Read the model definition and answer for the solid it produces. Units are mm, in the model's axes. Face numbers are marked on the shaded views. Give positions to 0.01 mm unless a question says otherwise; leave off trailing zeros. Loops run counter-clockwise (first coordinate to the right, second up) from the corner with the lowest first, then second, coordinate; pieces in that order, holes last. Notation, with made-up numbers: (43, 65.5) -> (99, 65.5) arc R7 ccw to (99, 71.5) -> close; hole circle Ø2 at (8, 66.25). An arc over 180 degrees is marked (long way). Return JSON: item names as keys, results as strings. Group by question number.
Autodesk Inventor part; units mm, degrees
ref_plane "YZ Plane" through (0, 0, 0) normal (1, 0, 0) x (0, 1, 0)
ref_plane "XZ Plane" through (0, 0, 0) normal (0, 1, 0) x (-1, 0, 0)
ref_plane "XY Plane" through (0, 0, 0) normal (0, 0, 1) x (1, 0, 0)
sketch "Sketch1" plane through (0, 0, 0) normal (0, 0, 1) x (1, 0, 0)
  line L0 (-66.75, 41.75) -> (66.75, 41.75)
  line L1 (66.75, 41.75) -> (66.75, -41.75)
  line L2 (66.75, -41.75) -> (-66.75, -41.75)
  line L3 (-66.75, -41.75) -> (-66.75, 41.75)
  line L4 (-66.75, 41.75) -> (66.75, -41.75) construction
  line L5 (66.75, 41.75) -> (-66.75, -41.75) construction
  circle A0 centre (-63.75, 38.75) radius 1.5
  circle A1 centre (63.75, 38.75) radius 1.5
  circle A2 centre (63.75, -38.75) radius 1.5
  circle A3 centre (-63.75, -38.75) radius 1.5
  point P0 (0, 0)
  dimension "d0" = 133.5
  dimension "d1" = 83.5
  dimension "d2" = 3
  dimension "d3" = 3
  dimension "d4" = 3
  dimension "d5" = 3
  dimension "d6" = 3
  dimension "d7" = 3
  dimension "d8" = 3
  dimension "d9" = 3
  dimension "d10" = 3
  dimension "d11" = 3
  dimension "d12" = 3
  dimension "d13" = 3
extrude "Extrusion1" add sketch "Sketch1" along normal blind 1.75
fillet "Fillet1" radius 3 4 edges at (66.75, 41.75, 0.875) (-66.75, 41.75, 0.875) (66.75, -41.75, 0.875) (-66.75, -41.75, 0.875)
sketch "Sketch2" plane through (0, 0, 1.75) normal (0, 0, 1) x (1, 0, 0)
  line L0 (-59.5, 37.75) -> (59.5, 37.75)
  line L1 (59.5, 37.75) -> (59.5, -39.75)
  line L2 (59.5, -39.75) -> (-59.5, -39.75)
  line L3 (-59.5, -39.75) -> (-59.5, 37.75)
  line L4 (-59.5, 37.75) -> (59.5, -39.75) construction
  line L5 (59.5, 37.75) -> (-59.5, -39.75) construction
  line L6 (63.75, 41.75) -> (-63.75, 41.75)
  point P0 (0, 0)
  point P1 (0, -1)
  dimension "d17" = 0
  dimension "d19" = 77.5
  dimension "d20" = 4
  dimension "d21" = 119
extrude "Extrusion2" add sketch "Sketch2" along normal blind 4.65
sketch "Sketch3" plane through (0, 0, 0) normal (0, 0, -1) x (-1, 0, 0)
  line L0 (66.75, -7.5) -> (58.75, -7.5)
  line L1 (58.75, -7.5) -> (58.75, 7.5)
  line L2 (58.75, 7.5) -> (66.75, 7.5)
  line L3 (66.75, 7.5) -> (66.75, -7.5)
  line L4 (66.75, -7.5) -> (58.75, 7.5) construction
  line L5 (58.75, -7.5) -> (66.75, 7.5) construction
  line L6 (-66.75, -7.5) -> (-58.75, -7.5)
  line L7 (-58.75, -7.5) -> (-58.75, 7.5)
  line L8 (-58.75, 7.5) -> (-66.75, 7.5)
  line L9 (-66.75, 7.5) -> (-66.75, -7.5)
  line L10 (-66.75, -7.5) -> (-58.75, 7.5) construction
  line L11 (-58.75, -7.5) -> (-66.75, 7.5) construction
  line L12 (-66.75, -38.75) -> (-66.75, 38.75)
  line L13 (66.75, 38.75) -> (66.75, -38.75)
  point P0 (0, 0)
  point P1 (62.75, 0)
  point P2 (-62.75, 0)
  dimension "d24" = 8
  dimension "d25" = 15
  dimension "d26" = 8
  dimension "d27" = 15
  dimension "d28" = 0
  dimension "d29" = 0
  dimension "d30" = 0
  dimension "d31" = 0
extrude "Extrusion3" add sketch "Sketch3" along normal blind 6.25
fillet "Fillet2" radius 2 6 edges at (-62.75, 7.5, 0) (-58.75, 0, 0) (-62.75, -7.5, 0) (62.75, 7.5, 0) (58.75, 0, 0) (62.75, -7.5, 0)
fillet "Fillet3" radius 2 4 edges at (62.75, 7.5, -6.25) (62.75, -7.5, -6.25) (-62.75, 7.5, -6.25) (-62.75, -7.5, -6.25)
equation "\"d8\" = d6"
equation "\"d9\" = d7"
equation "\"d10\" = d7"
equation "\"d11\" = d6"
equation "\"d12\" = d6"
equation "\"d13\" = d6"
equation "\"d26\" = d24"
equation "\"d27\" = d25"
properties part number "Tela Led"
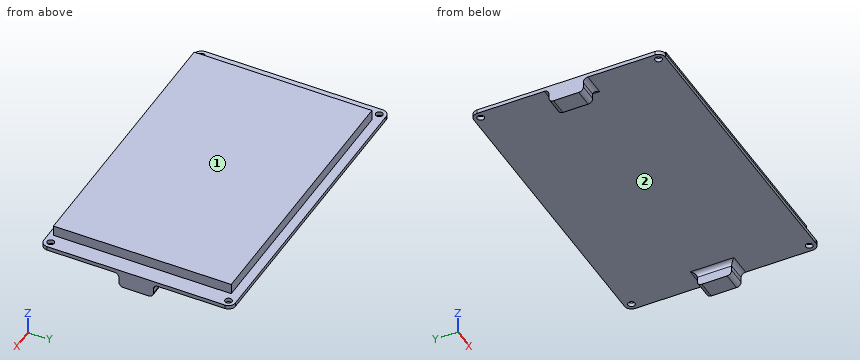
1. Section A-A on x = -13.5 is taken. Determine the outline of the cut face in (y, z), then the cut area to 4 significant figures.
2. Section B-B on y = -15.5 is taken. Determine the outline of the cut face in (x, z), then the cut area to 3 significant figures.
3. Straight lines are drawn through the part: line 1 (Y direction, x = -63.75, z = 0.9); line 2 (X direction, y = -2, z = -5.5). For each, find the intervals that lie inside material, in ascending order. Write a range as from..to.
4. Flat-ended cylindrical pins translate along their axes: pin 1 Ø5 at (y, z) = (-1, 4.5) entering from +X; pin 2 Ø2.5 at (x, z) = (-28, 4.5) entering from -Y; pin 3 Ø1.1 at (x, z) = (-63, -2.5) entering from +Y; pin 4 Ø2.5 at (x, y) = (63.75, -38.75) entering from -Z. Find the tip coordinate at first contact, or state that the pin passes through.
5. Determine the mould class of the marked faces 1 and 2 for opening direction X: pulls with the +X half, pulls with the -X half, needs draft (parallel to the pull), parting line crosses it, or undercut.
Completed:
{
 "1": {"outline": "(-41.75, 0) -> (41.75, 0) -> (41.75, 1.75) -> (37.75, 1.75) -> (37.75, 6.4) -> (-39.75, 6.4) -> (-39.75, 1.75) -> (-41.75, 1.75) -> close", "area": "506.5 mm²"},
 "2": {"outline": "(-66.75, 0) -> (66.75, 0) -> (66.75, 1.75) -> (59.5, 1.75) -> (59.5, 6.4) -> (-59.5, 6.4) -> (-59.5, 1.75) -> (-66.75, 1.75) -> close", "area": "787 mm²"},
 "3": {"line 1": "y = -41.75..-40.25, -37.25..37.25, 40.25..41.75", "line 2": "x = -66.75..-58.75, 58.75..66.75"},
 "4": {"pin 1": "stops at x = 59.5", "pin 2": "stops at y = -39.75", "pin 3": "stops at y = 7.5", "pin 4": "passes through"},
 "5": {"face 1": "needs draft", "face 2": "undercut"}
}
